Source: three-view drawing plus pictorial views. Frame: mm from the lowest corner of the part. A direction names the side the tool comes from. Coordinates: 2 decimals unless noted, no trailing zeros. Order: outer loops, then holes, each group sorted by start corner. A loop starts at its lowest first (then second) coordinate and runs counter-clockwise, first axis right, second up. Notation, with made-up numbers: (-5.5, -37.75) - (24.5, -37.75) arc R30 ccw to (24.5, -2.75) - close; hole circle Ø7 at (87, 10.5). An arc over 180 degrees is marked (long way). One line per question, with ' | ' between items.
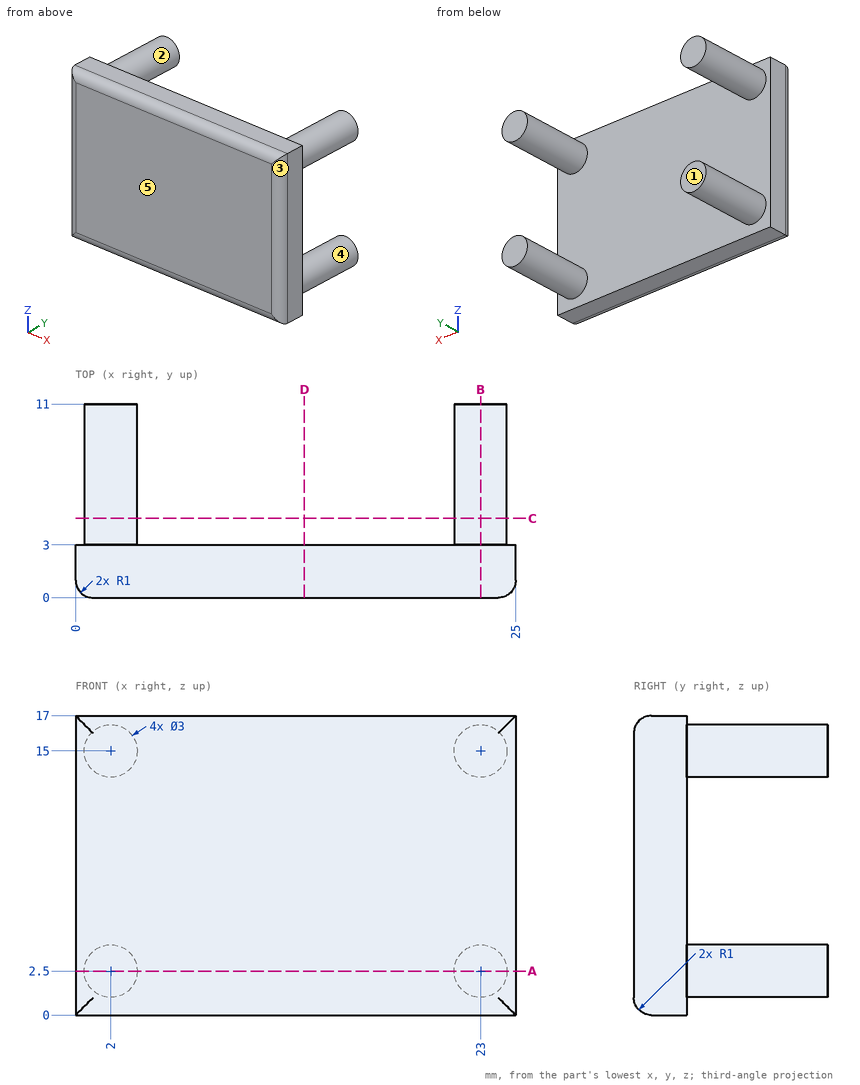
(1) Cut plane A-A (z = 2.5). Return the cut outline in (x, y).
Taken from the geometry:
outline: (0, 1) arc R1 ccw to (1, 0) - (24, 0) arc R1 ccw to (25, 1) - (25, 3) - (24.5, 3) - (24.5, 11) - (21.5, 11) - (21.5, 3) - (3.5, 3) - (3.5, 11) - (0.5, 11) - (0.5, 3) - (0, 3) - close
(2) Cut plane B-B (x = 23). Return the cut outline in (y, z), and give its area (3 significant figures).
Taken from the geometry:
outline: (0, 1) arc R1 ccw to (1, 0) - (3, 0) - (3, 1) - (11, 1) - (11, 4) - (3, 4) - (3, 13.5) - (11, 13.5) - (11, 16.5) - (3, 16.5) - (3, 17) - (1, 17) arc R1 ccw to (0, 16) - close | area: 98.6 mm²
(3) Material intervals for L1, parallel to Y at x = 10.75, z = 7.5; L2, parallel to X at y = 10.5, z = 15; L3, parallel to X at y = 6.75, z = 2, sorted ascending. Write a range as from..to.
Taken from the geometry:
L1: y = 0..3 | L2: x = 0.5..3.5, 21.5..24.5 | L3: x = 0.59..3.41, 21.59..24.41
(4) Cut plane D-D (x = 13). Return the cut outline in (y, z), and give its area (3 significant figures).
Taken from the geometry:
outline: (0, 1) arc R1 ccw to (1, 0) - (3, 0) - (3, 17) - (1, 17) arc R1 ccw to (0, 16) - close | area: 50.6 mm²
(5) Set-up query: the marked faces 4 and 5. Return all of +Z, -Z, +X, -X, +Y, -Y with unobstructed straight access to the full face (end or side cutting, diameter ignored); none if empty.
Taken from the geometry:
face 4: +Y | face 5: +Z, -Z, +X, -X, -Y
(6) Cut plane C-C (y = 4.5). Return the cut outline in (x, z).
Taken from the geometry:
outline: circle Ø3 at (2, 2.5); circle Ø3 at (2, 15); circle Ø3 at (23, 2.5); circle Ø3 at (23, 15)
(7) Pin query (flat end, axial travel): P1, Ø10, axis at x = 11, z = 2, coming from the +Y side; P2, Ø5, axis at y = 6, z = 4, coming from the +X side. Return the tip coordinate at first contact, or that it passes through.
Taken from the geometry:
P1: stops at y = 3 | P2: stops at x = 24.5
(8) Pull-direction query (X, two-part tool) for the marked faces 1, 2 and 3; classes: pulls with the +X half, pulls with the -X half, needs draft (parallel to the pull), parting line crosses it, or undercut.
Taken from the geometry:
face 1: needs draft | face 2: undercut | face 3: pulls with the +X half
